CAD build for the part. Positions are in the model's coordinates, mm. Give positions to 0.01 mm unless a question says otherwise; leave off trailing zeros. Write each loop counter-clockwise with the first axis right and the second up, starting at its lowest first coordinate (ties: lowest second). Pieces come first, ordered by that corner, then holes. Notation, with made-up numbers: (86, 33) -> (111, 33) arc R25 ccw to (111, 45) -> close; hole circle Ø1 at (56, 67). An arc over 180 degrees is marked (long way). Answer in a Markdown table with one row per item. Add a question column.
```python
from build123d import *

# Parameters (mm, degrees)
F0_W        = 76.2
F0_H        = 25.4
F1_DEPTH    = 1.27
F2_T1_DEPTH = 132.64003455
F3_R        = 0.508
F4_DEPTH    = 1.27
F5_R        = 0.508
F6_DEPTH    = 1.27
F7_R        = 1.27
F8_DEPTH    = 25.4


# Not quite as in the source:
# - a fillet or chamfer that OpenCascade refuses, or shapes differently, is made with other operations: its cross-section is extruded or revolved along the edge and cut away or added


with BuildPart() as f1:
    # F0 (on Front) → F1 (new body)
    with BuildSketch(Plane.XZ):
        with Locations((-28.6749217987, 43.1045838744)):
            Rectangle(F0_W, F0_H)
    extrude(amount=F1_DEPTH)

    # F2: fillet of radius 50.8 on 1 edges, made by hand

    # F2_s2 → F2_t1 (cut)
    with BuildSketch(Plane.YZ.offset(-94.9949390737)):
        with BuildLine():
            ThreePointArc((0, 30.4045838744), (-0.9515015625, 36.0129781215), (-1.27, 41.6925907843))
            Line((-1.27, 41.6925907843), (-2.286, 41.6925907843))
            Line((-2.286, 41.6925907843), (-2.286, 30.4045838744))
            Line((-2.286, 30.4045838744), (-1.27, 29.3885838744))
            ThreePointArc((-1.27, 29.3885838744), (-0.635, 29.3885838744), (-0.9906, 30.1788237362))
            Line((-0.9906, 30.1788237362), (0, 30.4045838744))
        make_face()
    extrude(amount=F2_T1_DEPTH, mode=Mode.SUBTRACT)

    # F3 (on face) → F4 (cut)
    with BuildSketch(Plane(origin=(-66.7749217987, 0, 0), x_dir=(0, -1, 0), z_dir=(-1, 0, 0))):
        with Locations((0.635, 44.3745838744)):
            Circle(F3_R)
    extrude(amount=-F4_DEPTH, mode=Mode.SUBTRACT)

    # F5 (on face) → F6 (cut)
    with BuildSketch(Plane.YZ.offset(9.4250782013)):
        with Locations((-0.635, 44.3745838744)):
            Circle(F5_R)
    extrude(amount=-F6_DEPTH, mode=Mode.SUBTRACT)

    # F7 (on face) → F8 (cut)
    with BuildSketch(Plane.XZ.offset(1.27)):
        with Locations((-28.6749217987, 54.2805838744)):
            Circle(F7_R)
    extrude(amount=-F8_DEPTH, mode=Mode.SUBTRACT)


solid = f1.part
```
Item 1: Slice it at C-C, the plane x = -54. List the corners of the cut face in (y, z), then the cut area to 3 significant figures.
Item 2: Probe L1, parallel to Y at x = 0.5, z = 41.5; L2, parallel to X at y = -0.6, z = 54.75; L3, parallel to Y at x = 0, z = 36.5. List the from-to ranges inside material, lowest first. Write a range as from..to.
Item 3: Slice it at B-B, the plane y = -0.95. List the corners of the cut face in (x, z).
Item 4: Slice it at D-D, the plane z = 35.75. List the corners of the cut face in (x, y).
Item 5: Slice it at A-A, the plane x = -29. List the corners of the cut face in (y, z).
Item 6: Mould opens along X. For faces 1 (the face through (-27.464, -0.644, 54.662)), 2 (the face through (-66.775, -1, 46)), 3 (the face through (-29, 0, 43)) say: released by +X, released by -X, zero draft, split by the parting line, or undercut.
Answer key:
| question | item | result |
|---|---|---|
| 1 | outline | (-1.27, 41.69) arc R50.8 ccw to (0, 30.4) -> (0, 55.8) -> (-1.27, 55.8) -> close |
| 1 | area | 27.5 mm² |
| 2 | L1 | y = -1.27..0 |
| 2 | L2 | x = -66.77..-29.85, -27.49..9.43 |
| 2 | L3 | y = -1..0 |
| 3 | outline | (-66.77, 36) -> (9.43, 36) -> (9.43, 43.98) -> (8.16, 43.98) -> (8.16, 44.77) -> (9.43, 44.77) -> (9.43, 55.8) -> (-66.77, 55.8) -> (-66.77, 44.77) -> (-65.5, 44.77) -> (-65.5, 43.98) -> (-66.77, 43.98) -> close; hole circle Ø2.54 at (-28.67, 54.28) |
| 4 | outline | (-66.77, -0.92) -> (9.43, -0.92) -> (9.43, 0) -> (-66.77, 0) -> close |
| 5 | outline | (-1.27, 41.69) arc R50.8 ccw to (0, 30.4) -> (0, 53.05) -> (-1.27, 53.05) -> close; (-1.27, 55.51) -> (0, 55.51) -> (0, 55.8) -> (-1.27, 55.8) -> close |
| 6 | face 1 | undercut |
| 6 | face 2 | released by -X |
| 6 | face 3 | zero draft |
